from build123d import *

# Parameters (mm, degrees)
F2_DEPTH = 50.8
F1_R     = 10.802579
F1_R_2   = 10.017442
F3_DEPTH = 25.4


with BuildPart() as f2:
    # F0 (on Front) → F2 (new body)
    with BuildSketch(Plane.XZ):
        with BuildLine():
            ThreePointArc((-84.818284, 4.49832), (-74.075205, 12.619594), (-61.718, 17.973872))
            ThreePointArc((-61.718, 17.973872), (-105.003657, 65.638275), (-84.818284, 4.49832))
        make_face()
        with BuildLine():
            ThreePointArc((-33.519126, 19.040262), (-47.686065, 20.292057), (-61.718, 17.973872))
            ThreePointArc((-61.718, 17.973872), (-74.075205, 12.619594), (-84.818284, 4.49832))
            ThreePointArc((-84.818284, 4.49832), (-67.706115, -88.386562), (11.071378, -36.285371))
            ThreePointArc((11.071378, -36.285371), (5.655705, -12.12097), (-9.555264, 7.420632))
            ThreePointArc((-9.555264, 7.420632), (-20.844259, 14.65953), (-33.519126, 19.040262))
        make_face()
        with BuildLine():
            ThreePointArc((-9.555264, 7.420632), (5.818639, 69.648031), (-33.519126, 19.040262))
            ThreePointArc((-33.519126, 19.040262), (-20.844259, 14.65953), (-9.555264, 7.420632))
        make_face()
    extrude(amount=F2_DEPTH)

    # F1 (on Front) → F3 (cut)
    with BuildSketch(Plane.XZ):
        with Locations((-75.122081, -19.301618)):
            Circle(F1_R)
        with Locations((-25.931325, -18.290848)):
            Circle(F1_R_2)
    extrude(amount=-F3_DEPTH, mode=Mode.SUBTRACT)


solid = f2.part
Verification items for the finished model (mm, model axes). Give positions to 0.01 mm unless a question says otherwise; leave off trailing zeros. Order: outer loops, then holes, each group sorted by start corner. A loop starts at its lowest first (then second) coordinate and runs counter-clockwise, first axis right, second up. Notation, with made-up numbers: M 19.5,87 L 31.5,87 A19 ccw 31.5,117 Z; hole C -24.5,-11.5 d7. An arc over 180 degrees is marked long. Use one line per item in the form item = value. Start each with the question number.
Q1. Scan lines: line 1 along X through (y, z) = (-31, -35); line 2 along X through (y, z) = (-14, 34.5); line 3 along X through (y, z) = (-8, 30.5). Record each from-to range of solid material in increasing order. Write a range as [from, to].
Q2. Section check A-A (x = -1). Enter the section's corners in (y, z), then the cut area to 3 significant figures.
Q3. Section check B-B (z = 54). Enter the section's corners in (x, y), then the cut area to 3 significant figures.
Q4. Section check D-D (x = -19). Enter the section's corners in (y, z).
Q5. Go/stop test with flat-tipped pins: pin 1 Ø12 at (x, y) = (-68, -26) entering from +Z; pin 2 Ø4 at (y, z) = (-12, 19) entering from -X; pin 3 Ø6 at (x, y) = (-3.5, -34) entering from -Z. Record where each tip stops, or that it passes through.
Q6. Section check C-C (y = -31.5). Enter the section's corners in (x, z).
Q7. Mould release check, pull along Z, two halves, no side actions. Record for faces 1 (the flat face through (-50, 0, -9)), 2 (the cylindrical face through (-103.91, -25.04, 66.25)): +Z half, -Z half, draft (parallel to the pull), parting line (faces both ways), or undercut.
Evaluation:
q1.line_1 = [-102.15, 11.06]
q1.line_2 = [-121.22, -55.62], [-40.75, 23.79]
q1.line_3 = [-120.64, -56.2], [-39.78, 22.83]
q2.outline = M -50.8,-71.23 L 0,-71.23 L 0,-1.34 L -50.8,-1.34 Z; M -50.8,8.27 L 0,8.27 L 0,72.07 L -50.8,72.07 Z
q2.area = 6,790 mm2
q3.outline = M -116.73,-50.8 L -60.11,-50.8 L -60.11,0 L -116.73,0 Z; M -38.18,-50.8 L 21.22,-50.8 L 21.22,0 L -38.18,0 Z
q3.area = 5,890 mm2
q4.outline = M -50.8,-86.29 L 0,-86.29 L 0,71.19 L -50.8,71.19 Z
q5.pin_1 = 66.79
q5.pin_2 = -117.06
q5.pin_3 = -77.28
q6.outline = M -84.82,4.5 A56.62 ccw long 11.07,-36.29 A56.62 ccw -9.56,7.42 A32.76 ccw long -33.52,19.04 A56.62 ccw -61.72,17.97 A32.91 ccw long Z
q7.face_1 = draft
q7.face_2 = undercut
